The listing builds one solid part. Answer for the finished solid, in the listing's coordinates (mm). Face numbers are marked on the shaded views. A direction names the side the tool comes from. Give positions to 0.01 mm unless a question says otherwise; leave off trailing zeros. Write each loop counter-clockwise with the first axis right and the second up, starting at its lowest first coordinate (ties: lowest second). Pieces come first, ordered by that corner, then holes. Notation, with made-up numbers: (-9, 67.25) - (37, 67.25) arc R24 cw to (37, 87.25) - close; hole circle Ø4 at (73.5, -36). An arc over 180 degrees is marked (long way). One line per item, written item: value. Start each with the question number.
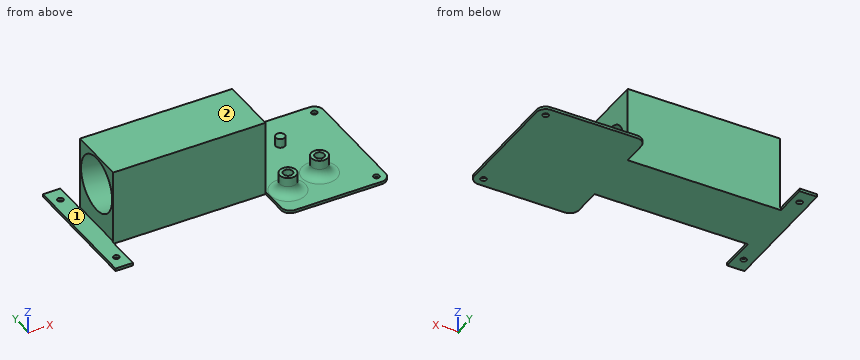
from build123d import *

# Parameters (mm, degrees)
ESQUISSE1_W             = 140
ESQUISSE1_H             = 70
BOSS_EXTRU_1_DEPTH      = 1.5
ESQUISSE2_R             = 1.6
ENL_V_MAT_EXTRU_2_DEPTH = 1.5
ESQUISSE2_4_R           = 2.5
BOSS_EXTRU_2_DEPTH      = 5
BOSS_EXTRU_3_DEPTH      = 40
ESQUISSE11_R            = 4.5
ESQUISSE11_R_2          = 2.6
BOSS_EXTRU_4_DEPTH      = 10
CONG_1_R                = 5
ESQUISSE14_W            = 83
ESQUISSE14_H            = 18
ESQUISSE14_H_2          = 20
ENL_V_MAT_EXTRU_3_DEPTH = 162.554944214
CONG_3_R                = 5
ESQUISSE17_W            = 1.5
ESQUISSE17_H            = 70
BOSS_EXTRU_5_DEPTH      = 10
ESQUISSE18_R            = 1.6
ENL_V_MAT_EXTRU_4_DEPTH = 162.554944239
ESQUISSE22_W            = 1.5
ESQUISSE22_H            = 18
ESQUISSE22_H_2          = 20
ENL_V_MAT_EXTRU_5_DEPTH = 0.5


with BuildPart() as part:
    # Esquisse1 → Boss.-Extru.1 (new body)
    with BuildSketch(Plane.XY):
        with Locations((70, -35)):
            Rectangle(ESQUISSE1_W, ESQUISSE1_H)
    extrude(amount=BOSS_EXTRU_1_DEPTH)

    # Esquisse2 → Enlèv. mat.-Extru.2 (cut)
    with BuildSketch(Plane.XY.offset(1.5)):
        with Locations((135, -5)):
            Circle(ESQUISSE2_R)
        with Locations((135, -65)):
            Circle(ESQUISSE2_R)
    extrude(amount=-ENL_V_MAT_EXTRU_2_DEPTH, mode=Mode.SUBTRACT)

    # Esquisse2<4> → Boss.-Extru.2 (add)
    with BuildSketch(Plane.XY.offset(1.5)):
        with Locations((108, -20)):
            Circle(ESQUISSE2_4_R)
    extrude(amount=BOSS_EXTRU_2_DEPTH)

    # Esquisse2<5> → Boss.-Extru.3 (add)
    with BuildSketch(Plane.XY.offset(1.5)):
        Polygon((83, -18), (0, -18), (0, -50), (7.5, -50), (75, -50), (76.464784117, -50), (83, -50), (83, -45), align=None)
    extrude(amount=BOSS_EXTRU_3_DEPTH)

    # Esquisse11 → Boss.-Extru.4 (add)
    # profile 1 of 2: a face of its own
    with BuildSketch(Plane.XY.offset(1.5)):
        with Locations((113, -49)):
            Circle(ESQUISSE11_R)
        with Locations((113, -49)):
            Circle(ESQUISSE11_R_2, mode=Mode.SUBTRACT)
    # profile 2 of 2: a face of its own
    with BuildSketch(Plane.XY.offset(1.5)):
        with Locations((93, -54)):
            Circle(ESQUISSE11_R)
        with Locations((93, -54)):
            Circle(ESQUISSE11_R_2, mode=Mode.SUBTRACT)
    extrude(amount=BOSS_EXTRU_4_DEPTH)

    # Congé1
    cong_1_edges = [part.edges().sort_by_distance(p)[0] for p in [
        (108.5, -49, 1.5),
        (88.5, -54, 1.5),
    ]]
    fillet(cong_1_edges, radius=CONG_1_R)

    # Esquisse14 → Enlèv. mat.-Extru.3 (cut, through all)
    with BuildSketch(Plane.XY.offset(1.5)):
        with Locations((41.5, -9)):
            Rectangle(ESQUISSE14_W, ESQUISSE14_H)
        with Locations((41.5, -60)):
            Rectangle(ESQUISSE14_W, ESQUISSE14_H_2)
    extrude(amount=-ENL_V_MAT_EXTRU_3_DEPTH, mode=Mode.SUBTRACT)

    # Congé3
    cong_3_edges = [part.edges().sort_by_distance(p)[0] for p in [
        (83, 0, 0.75),
        (140, 0, 0.75),
        (140, -70, 0.75),
        (83, -70, 0.75),
    ]]
    fillet(cong_3_edges, radius=CONG_3_R)

    # Enlèvement de matière-Lissage1: read off the stored shape, not the designer's step
    # Enlèvement de matière-Lissage1: loft between two sections, ruled curve by curve
    enl_vement_de_mati_re_lissage1_from = [
        Edge.make_bspline([(0, -35.358936945, 10.061683817), (0, -34.736507104, 10.005061444), (0, -34.071276467, 9.983471322), (0, -32.656620792, 10.043511569), (0, -31.906986183, 10.125212836), (0, -30.336715689, 10.432215403), (0, -29.515853558, 10.657740433), (0, -27.835171711, 11.295881241), (0, -26.97522752, 11.708928876), (0, -25.273092172, 12.759040897), (0, -24.43107638, 13.396695447), (0, -22.846227272, 14.910682395), (0, -22.104033135, 15.787505474), (0, -20.813231902, 17.754778804), (0, -20.26561628, 18.845205387), (0, -19.446047462, 21.166299645), (0, -19.174928563, 22.396203373), (0, -18.948439072, 24.885922737), (0, -18.993175694, 26.144559807), (0, -19.380457825, 28.575441159), (0, -19.722320583, 29.746783491), (0, -20.636945499, 31.91468419), (0, -21.20873673, 32.91104037), (0, -22.494376602, 34.686155378), (0, -23.207508016, 35.465281495), (0, -24.692213453, 36.805300064), (0, -25.463508496, 37.366741349), (0, -27.001451353, 38.297680084), (0, -27.768143671, 38.667624764), (0, -29.257240332, 39.252937618), (0, -29.979826835, 39.468566674), (0, -31.360426607, 39.782890995), (0, -32.018633214, 39.88169381), (0, -33.263492896, 39.994938556), (0, -33.928723533, 40.016528678), (0, -35.343379208, 39.956488431), (0, -36.093013817, 39.874787164), (0, -37.663284311, 39.567784597), (0, -38.484146442, 39.342259567), (0, -40.164828289, 38.704118759), (0, -41.02477248, 38.291071124), (0, -42.726907828, 37.240959103), (0, -43.56892362, 36.603304553), (0, -45.153772728, 35.089317605), (0, -45.895966865, 34.212494526), (0, -47.186768098, 32.245221196), (0, -47.73438372, 31.154794613), (0, -48.553952538, 28.833700355), (0, -48.825071437, 27.603796627), (0, -49.051560928, 25.114077263), (0, -49.006824306, 23.855440193), (0, -48.619542175, 21.424558841), (0, -48.277679417, 20.253216509), (0, -47.363054501, 18.08531581), (0, -46.79126327, 17.08895963), (0, -45.505623398, 15.313844622), (0, -44.792491984, 14.534718505), (0, -43.307786547, 13.194699936), (0, -42.536491504, 12.633258651), (0, -40.998548647, 11.702319916), (0, -40.231856329, 11.332375236), (0, -38.742759668, 10.747062382), (0, -38.020173165, 10.531433326), (0, -36.639573393, 10.217109005), (0, -35.981366786, 10.11830619), (0, -35.358936945, 10.061683817)], [0, 0, 0, 0, 0.03125, 0.03125, 0.0625, 0.0625, 0.09375, 0.09375, 0.125, 0.125, 0.15625, 0.15625, 0.1875, 0.1875, 0.21875, 0.21875, 0.25, 0.25, 0.28125, 0.28125, 0.3125, 0.3125, 0.34375, 0.34375, 0.375, 0.375, 0.40625, 0.40625, 0.4375, 0.4375, 0.46875, 0.46875, 0.5, 0.5, 0.53125, 0.53125, 0.5625, 0.5625, 0.59375, 0.59375, 0.625, 0.625, 0.65625, 0.65625, 0.6875, 0.6875, 0.71875, 0.71875, 0.75, 0.75, 0.78125, 0.78125, 0.8125, 0.8125, 0.84375, 0.84375, 0.875, 0.875, 0.90625, 0.90625, 0.9375, 0.9375, 0.96875, 0.96875, 1, 1, 1, 1], 3),
    ]
    enl_vement_de_mati_re_lissage1_to = [
        Edge.make_bspline([(83, -36.978683165, 4.157601006), (83, -36.46441654, 4.075155874), (83, -35.912574895, 4.019404171), (83, -34.733027399, 3.988933266), (83, -34.105143284, 4.014261099), (83, -32.782184956, 4.18027026), (83, -32.086909931, 4.321124739), (83, -30.653339337, 4.756165981), (83, -29.914915742, 5.050704715), (83, -28.440098529, 5.827037097), (83, -27.703817174, 6.30933137), (83, -26.300151244, 7.477991211), (83, -25.633270194, 8.16480105), (83, -24.448315736, 9.727029605), (83, -23.931067977, 10.602484983), (83, -23.117787224, 12.485655838), (83, -22.82249127, 13.492783585), (83, -22.492710742, 15.549850084), (83, -22.458382278, 16.598815077), (83, -22.642231037, 18.641841677), (83, -22.85989188, 19.635114611), (83, -23.497113975, 21.489467093), (83, -23.915879492, 22.35032337), (83, -24.883881149, 23.899199305), (83, -25.432500118, 24.587483568), (83, -26.590728024, 25.785935025), (83, -27.200073831, 26.296542663), (83, -28.425809001, 27.15791298), (83, -29.04220995, 27.509050012), (83, -30.246974936, 28.080293485), (83, -30.835475596, 28.300627173), (83, -31.965435919, 28.640407161), (83, -32.50705021, 28.759953862), (83, -33.53558346, 28.924844126), (83, -34.087425105, 28.980595829), (83, -35.266972601, 29.011066734), (83, -35.894856716, 28.985738901), (83, -37.217815044, 28.81972974), (83, -37.913090069, 28.678875261), (83, -39.346660663, 28.243834019), (83, -40.085084258, 27.949295285), (83, -41.559901471, 27.172962903), (83, -42.296182826, 26.69066863), (83, -43.699848756, 25.522008789), (83, -44.366729806, 24.83519895), (83, -45.551684264, 23.272970395), (83, -46.068932023, 22.397515017), (83, -46.882212776, 20.514344162), (83, -47.17750873, 19.507216415), (83, -47.507289258, 17.450149916), (83, -47.541617722, 16.401184923), (83, -47.357768963, 14.358158323), (83, -47.14010812, 13.364885389), (83, -46.502886025, 11.510532907), (83, -46.084120508, 10.64967663), (83, -45.116118851, 9.100800695), (83, -44.567499882, 8.412516432), (83, -43.409271976, 7.214064975), (83, -42.799926169, 6.703457337), (83, -41.574190999, 5.84208702), (83, -40.95779005, 5.490949988), (83, -39.753025064, 4.919706515), (83, -39.164524404, 4.699372827), (83, -38.034564081, 4.359592839), (83, -37.49294979, 4.240046138), (83, -36.978683165, 4.157601006)], [0, 0, 0, 0, 0.03125, 0.03125, 0.0625, 0.0625, 0.09375, 0.09375, 0.125, 0.125, 0.15625, 0.15625, 0.1875, 0.1875, 0.21875, 0.21875, 0.25, 0.25, 0.28125, 0.28125, 0.3125, 0.3125, 0.34375, 0.34375, 0.375, 0.375, 0.40625, 0.40625, 0.4375, 0.4375, 0.46875, 0.46875, 0.5, 0.5, 0.53125, 0.53125, 0.5625, 0.5625, 0.59375, 0.59375, 0.625, 0.625, 0.65625, 0.65625, 0.6875, 0.6875, 0.71875, 0.71875, 0.75, 0.75, 0.78125, 0.78125, 0.8125, 0.8125, 0.84375, 0.84375, 0.875, 0.875, 0.90625, 0.90625, 0.9375, 0.9375, 0.96875, 0.96875, 1, 1, 1, 1], 3),
    ]
    enl_vement_de_mati_re_lissage1 = Solid(Shell([*[Face.make_surface_from_curves(enl_vement_de_mati_re_lissage1_from[k], enl_vement_de_mati_re_lissage1_to[k]) for k in range(1)], Face(Wire(enl_vement_de_mati_re_lissage1_from)), Face(Wire(enl_vement_de_mati_re_lissage1_to))]))
    add(enl_vement_de_mati_re_lissage1, mode=Mode.SUBTRACT)

    # Esquisse17 → Boss.-Extru.5 (add)
    with BuildSketch(Plane.ZY):
        with Locations((0.75, -35)):
            Rectangle(ESQUISSE17_W, ESQUISSE17_H)
    extrude(amount=BOSS_EXTRU_5_DEPTH)

    # Esquisse18 → Enlèv. mat.-Extru.4 (cut, through all)
    with BuildSketch(Plane.XY.offset(1.5)):
        with Locations((-5, -8)):
            Circle(ESQUISSE18_R)
        with Locations((-5, -62)):
            Circle(ESQUISSE18_R)
    extrude(amount=-ENL_V_MAT_EXTRU_4_DEPTH, mode=Mode.SUBTRACT)

    # Esquisse22 → Enlèv. mat.-Extru.5 (cut)
    with BuildSketch(Plane(origin=(0, 0, 0), x_dir=(0, 0, -1), z_dir=(1, 0, 0))):
        with Locations((-0.75, -9)):
            Rectangle(ESQUISSE22_W, ESQUISSE22_H)
        with Locations((-0.75, -60)):
            Rectangle(ESQUISSE22_W, ESQUISSE22_H_2)
    extrude(amount=-ENL_V_MAT_EXTRU_5_DEPTH, mode=Mode.SUBTRACT)


solid = part.part
Item 1: Straight lines are drawn through the part: line 1 along Y through (x, z) = (135, 0.4); line 2 along X through (y, z) = (-65, 1); line 3 along Y through (x, z) = (-5, 1.15). For each, find the intervals that lie inside material, in ascending order.
Item 2: Find section A-A on x = 113. Determine the outline of the cut face in (y, z).
Item 3: Find section B-B on y = -62. Give the number of separate pieces and of enclosed holes in the cut face, plus the area to 3 significant figures.
Item 4: For the marked faces 1 and 2, determine the directions among +Z, -Z, +X, -X, +Y, -Y from which every point of the face is accessible in a straight line to the end or side of a thin tool.
Item 5: Each of these flat-tipped pins is pushed along its axis until it touches: pin 1 Ø4.5 at (x, y) = (92, -52) entering from +Z; pin 2 Ø2.5 at (x, y) = (113.5, -48) entering from +Z; pin 3 Ø1 at (x, y) = (32.5, -46) entering from -Z; pin 4 Ø5.5 at (x, y) = (109, -19) entering from +Z. Where does it stop, or does it pass through?
Values:
1. line 1: -70 to -66.6, -63.4 to -6.6, -3.4 to 0
1. line 2: -10 to -0.5, 83 to 133.4, 136.6 to 140
1. line 3: -70 to -63.6, -60.4 to -9.6, -6.4 to 0
2. outline: (-70, 0) - (0, 0) - (0, 1.5) - (-39.5, 1.5) arc R5 cw to (-44.5, 6.5) - (-44.5, 11.5) - (-46.4, 11.5) - (-46.4, 1.5) - (-51.6, 1.5) - (-51.6, 11.5) - (-53.5, 11.5) - (-53.5, 6.5) arc R5 cw to (-58.5, 1.5) - (-70, 1.5) - close
3. separate pieces: 3
3. enclosed holes: 0
3. area: 96.2 mm^2
4. face 1: +Z, -X, +Y, -Y
4. face 2: +Z, +X, -X, +Y, -Y
5. pin 1: z = 11.5
5. pin 2: z = 1.5
5. pin 3: z = 0
5. pin 4: z = 6.5
